Part model, mm, in its own coordinate system. Face numbers are marked on the shaded views. A direction names the side the tool comes from. Give positions to 0.01 mm unless a question says otherwise; leave off trailing zeros. Write item = value, one per line. Start each with the question number.
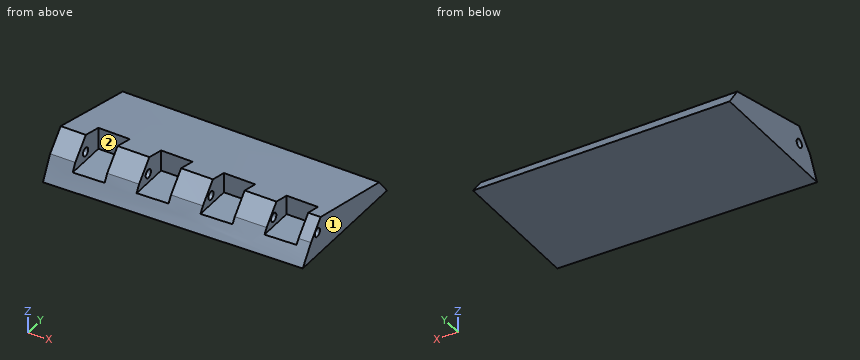
from build123d import *

# Parameters (mm, degrees)
F5_DEPTH  = 228.6
F7_W      = 27.94
F7_H      = 27.94
F8_DEPTH  = 25.4
F13_DEPTH = 609.6
F15_W     = 27.94
F15_H     = 27.94
F16_DEPTH = 25.4
F21_DEPTH = 50.8


with BuildPart() as f3:
    # F0 (on Right) → F3 section 0
    with BuildSketch(Plane.YZ):
        Polygon((-127, 0), (0, 0), (-11.19021, 15.666293), (-101.271398, 36.647938), (-116.657943, 20.142378), align=None)
    # F2 (on offset) → F3 section 1
    with BuildSketch(Plane.YZ.offset(228.6)):
        Polygon((-122.475073, 0), (0, 0), (-11.412238, 14.267517), (-96.457832, 32.171853), (-110.445596, 16.785316), align=None)
    loft()

    # F4 (on offset) → F5 (cut)
    with BuildSketch(Plane.YZ.offset(228.6)):
        with BuildLine():
            ThreePointArc((-97.416677, 20.708883), (-105.011268, 20.69831), (-97.41667, 20.701834))
            ThreePointArc((-97.41667, 20.701834), (-97.416672, 20.705359), (-97.416677, 20.708883))
        make_face()
    extrude(amount=-F5_DEPTH, mode=Mode.SUBTRACT)

    # F7 (on offset) → F8 (cut)
    with BuildSketch(Plane.XY.offset(16.9164)):
        with Locations((36.068, -96.52)):
            Rectangle(F7_W, F7_H)
        with Locations((91.948, -96.52)):
            Rectangle(F7_W, F7_H)
        with Locations((147.828, -96.52)):
            Rectangle(F7_W, F7_H)
        Polygon((203.708, -82.55), (189.738, -82.55), (189.738, -110.49), (217.678, -110.49), (217.678, -82.55), align=None)
    extrude(amount=F8_DEPTH, mode=Mode.SUBTRACT)

    # F9 (on face) + F10 (on face) + F11 (on face) + F12 (on face) → F13 (cut)
    with BuildSketch(Plane.XZ.offset(82.55)):
        Polygon((50.038, 31.635782), (22.098, 32.000567), (22.098, 16.9164), (50.038, 16.9164), align=None)
    with BuildSketch(Plane.XZ.offset(82.55)):
        Polygon((105.918, 30.898753), (77.978, 31.268528), (77.978, 16.9164), (105.918, 16.9164), align=None)
    with BuildSketch(Plane.XZ.offset(82.55)):
        Polygon((161.798, 30.151425), (133.858, 30.526404), (133.858, 16.9164), (161.798, 16.9164), align=None)
    with BuildSketch(Plane.XZ.offset(82.55)):
        Polygon((217.678, 29.393352), (189.738, 29.773761), (189.738, 16.9164), (217.678, 16.9164), align=None)
    extrude(amount=F13_DEPTH, mode=Mode.SUBTRACT)

    # F15 (on offset) → F16 (cut)
    with BuildSketch(Plane.XY.offset(12.7)):
        with Locations((36.068, -96.52)):
            Rectangle(F15_W, F15_H)
        with Locations((91.948, -96.52)):
            Rectangle(F15_W, F15_H)
        with Locations((147.828, -96.52)):
            Rectangle(F15_W, F15_H)
        with Locations((203.708, -96.52)):
            Rectangle(F15_W, F15_H)
    extrude(amount=F16_DEPTH, mode=Mode.SUBTRACT)

    # F17 (on face) + F18 (on face) + F19 (on face) + F20 (on face) → F21 (cut)
    with BuildSketch(Plane.XZ.offset(82.55)):
        Polygon((50.038, 31.635782), (22.098, 32.000567), (22.098, 12.7), (50.038, 12.7), align=None)
    with BuildSketch(Plane.XZ.offset(82.55)):
        Polygon((105.918, 30.898753), (77.978, 31.268528), (77.978, 12.7), (105.918, 12.7), align=None)
    with BuildSketch(Plane.XZ.offset(82.55)):
        Polygon((161.798, 30.151425), (133.858, 30.526404), (133.858, 12.7), (161.798, 12.7), align=None)
    with BuildSketch(Plane.XZ.offset(82.55)):
        Polygon((217.678, 29.393352), (189.738, 29.773761), (189.738, 12.7), (217.678, 12.7), align=None)
    extrude(amount=F21_DEPTH, mode=Mode.SUBTRACT)


solid = f3.part
Q1. Tool access for the marked faces 1 and 2: list every direction of +Z, -Z, +X, -X, +Y, -Y with a clear straight run to the whole face (end or side of a thin tool).
Q2. Probe line 1 along X through (y, z) = (-83, 13); line 2 along Z through (x, y) = (40, -111.5); line 3 along Y through (x, z) = (184.5, 3). List the from-to ranges inside material, lowest first.
Q3. Drop flat-ended pins along their axis: P1, Ø14, axis at x = 94.5, y = -105, coming from the +Z side; P2, Ø4, axis at x = 117.5, y = -41.5, coming from the -Z side; P3, Ø6, axis at y = -101.21, z = 20.7, coming from the -X side; P4, Ø5.5, axis at x = 149, z = 19, coming from the -Y side. Give the stop position or say it passes through.
Working result:
q1.face_1 = +Z, -Z, +X, +Y, -Y
q1.face_2 = +Z, -Y
q2.line_1 = 0 to 22.1, 50.04 to 77.98, 105.92 to 133.86, 161.8 to 189.74, 217.68 to 228.6
q2.line_2 = 0 to 12.7
q2.line_3 = -121.33 to -2.35
q3.P1 = 12.7
q3.P2 = 0
q3.P3 = through
q3.P4 = -82.55
